```python
from build123d import *

# Parameters (mm, degrees)
SKETCH1_R               = 6
SKETCH1_R_2             = 1.5
BOSS_EXTRUDE1_DEPTH     = 2
SKETCH2_R               = 3
SKETCH2_R_2             = 1.5
BOSS_EXTRUDE2_DEPTH     = 8
CUT_EXTRUDE1_REACH      = 17.362
CUT_EXTRUDE1_END_RADIUS = 1.5
SKETCH3_R               = 1.2
SKETCH3_3_R             = 1.2
CUT_EXTRUDE2_DEPTH      = 2


with BuildPart() as part:
    # Sketch1 → Boss-Extrude1 (new body)
    with BuildSketch(Plane.XY):
        Circle(SKETCH1_R)
        Circle(SKETCH1_R_2, mode=Mode.SUBTRACT)
    extrude(amount=BOSS_EXTRUDE1_DEPTH)

    # Sketch2 → Boss-Extrude2 (add)
    with BuildSketch(Plane.XY.offset(2)):
        Circle(SKETCH2_R)
        Circle(SKETCH2_R_2, mode=Mode.SUBTRACT)
    extrude(amount=BOSS_EXTRUDE2_DEPTH)

    # Cut-Extrude1: up to this cylinder (the profile starts outside it)
    cut_extrude1_end = Plane(origin=(0, 0, 6.078366), z_dir=(0, 0, -1)) * Cylinder(CUT_EXTRUDE1_END_RADIUS, 38.724, mode=Mode.PRIVATE)
    # Sketch3 → Cut-Extrude1 (cut, up to the surface)
    with BuildSketch(Plane(origin=(0, 4, 0), x_dir=(-1, 0, 0), z_dir=(0, 1, 0)), mode=Mode.PRIVATE) as cut_extrude1_sk1:
        with Locations(Location((0.135733681, 6.078365877, 0), (0, 0, 90))):
            Circle(SKETCH3_R)
    cut_extrude1_tool1 = extrude(cut_extrude1_sk1.sketch, amount=-CUT_EXTRUDE1_REACH, mode=Mode.PRIVATE) - cut_extrude1_end
    add(cut_extrude1_tool1.solids().sort_by_distance((-0.135734, 4, 6.078366))[0], mode=Mode.SUBTRACT)

    # Sketch3_3 → Cut-Extrude2 (cut)
    with BuildSketch(Plane(origin=(0, 4, 0), x_dir=(-1, 0, 0), z_dir=(0, 1, 0))):
        Polygon((-2.173667395, 6.078365877), (-1.018966857, 4.078365877), (1.29043422, 4.078365877), (2.445134758, 6.078365877), (1.29043422, 8.078365877), (-1.018966857, 8.078365877), align=None)
        with Locations(Location((0.135733681, 6.078365877, 0), (0, 0, 90))):
            Circle(SKETCH3_3_R, mode=Mode.SUBTRACT)
    extrude(amount=-CUT_EXTRUDE2_DEPTH, mode=Mode.SUBTRACT)


solid = part.part
```
Model file for the job. Use its own axes, mm. A direction names the side the tool comes from. Give positions to 0.01 mm unless a question says otherwise; leave off trailing zeros. Write each loop counter-clockwise with the first axis right and the second up, starting at its lowest first coordinate (ties: lowest second). Pieces come first, ordered by that corner, then holes. Notation, with made-up numbers: (66, 7.25) -> (87, 7.25) arc R28 ccw to (87, 36.25) -> close; hole circle Ø11 at (86, 21.25). An arc over 180 degrees is marked (long way). Use CSV: the item, a comma, the result in double quotes. Start each with the question number.
1) Tool access for faces 5 (the flat face through (1.2, -1.2, 0)), 6 (the flat face through (1.46, 2.325, 7.315)), 7 (the cylindrical face through (-0.65, -2.93, 5.94)): list every direction of +Z, -Z, +X, -X, +Y, -Y with a clear straight run to the whole face (end or side of a thin tool).
2) Pin check, flat tips, straight feed: P1, Ø2, axis at x = 0.5, z = 8, coming from the +Y side; P2, Ø3, axis at x = -4, y = 2, coming from the -Z side; P3, Ø2, axis at x = -0.14, z = 6.08, coming from the +Y side; P4, Ø5, axis at y = -3.5, z = 1, coming from the -X side. Stop position of each tip, or through.
3) Cut at A-A on y = 0. List the corners of the cut face in (x, z).
4) Drill centre lines: L1, parallel to Y at x = 0, z = 8.25; L2, parallel to Z at x = 3.25, y = 2; L3, parallel to X at y = 1, z = 6. Where is each one in solid material? Low to high.
5) Cut at C-C on x = -0.75. List the corners of the cut face in (y, z), plus the area to 3 significant figures.
6) Cut at D-D on z = 2.25. List the corners of the cut face in (x, y).
7) Two-plate mould, pull along Y, no slides. Class faces 1 (the flat face through (1.3, -1.3, 10)), 2 (the flat face through (1, 2, 7)), 3 (the cylindrical face through (-6, 0, 1)), 4 (the cylindrical face through (-0.325, -1.464, 4.93)): released by +Y, released by -Y, zero draft, split by the parting line, or undercut.
8) Cut at B-B on z = 6.25. List the corners of the cut face in (x, y), plus the area to 3 significant figures.
Final values:
1,face 5,"-Z, +X, -X, +Y, -Y"
1,face 6,"+Y"
1,face 7,"+Z"
2,P1,"stops at y = 3"
2,P2,"stops at z = 0"
2,P3,"stops at y = -0.97"
2,P4,"stops at x = -5.92"
3,outline,"(-6, 0) -> (-1.5, 0) -> (-1.5, 10) -> (-3, 10) -> (-3, 2) -> (-6, 2) -> close; (1.5, 0) -> (6, 0) -> (6, 2) -> (3, 2) -> (3, 10) -> (1.5, 10) -> close"
4,L1,"y = -3 to -1.5, 1.5 to 3"
4,L2,"z = 0 to 2"
4,L3,"x = -2.83 to -1.33, 1.12 to 2.83"
5,outline,"(-5.95, 0) -> (-1.3, 0) -> (-1.3, 10) -> (-2.9, 10) -> (-2.9, 2) -> (-5.95, 2) -> close; (1.3, 0) -> (5.95, 0) -> (5.95, 2) -> (2.9, 2) -> (2.9, 4.08) -> (2, 4.08) -> (2, 5.05) -> (1.3, 5.05) -> close; (1.3, 7.11) -> (2, 7.11) -> (2, 8.08) -> (2.9, 8.08) -> (2.9, 10) -> (1.3, 10) -> close"
5,area,"39.2 mm2"
6,outline,"circle Ø6 at (0, 0); hole circle Ø3 at (0, 0)"
7,face 1,"zero draft"
7,face 2,"released by +Y"
7,face 3,"split by the parting line"
7,face 4,"undercut"
8,outline,"(-2.24, 2) arc R3 ccw (long way) to (2.07, 2.17) -> (2.07, 2) -> (1.05, 2) -> (1.05, 1.07) arc R1.5 cw (long way) to (-1.32, 0.71) -> (-1.32, 2) -> close"
8,area,"16.5 mm2"
